Geometry check sheet. Reference: the model listing, model coordinates, mm. Face numbers are marked on the shaded views. A direction names the side the tool comes from. Give positions to 0.01 mm unless a question says otherwise; leave off trailing zeros. Loops run counter-clockwise (first coordinate to the right, second up) from the corner with the lowest first, then second, coordinate; pieces in that order, holes last. Notation, with made-up numbers: (-13, -6) -> (33, -6) arc R9 ccw to (33, 4) -> close; hole circle Ø5 at (75, 16.25). An arc over 180 degrees is marked (long way). Answer as a JSON object with one key per item and string values.
from build123d import *

# Parameters (mm, degrees)
SKETCH1_W           = 10
SKETCH1_H           = 10
BOSS_EXTRUDE1_DEPTH = 5
CUT_EXTRUDE1_START  = 1.25
CUT_EXTRUDE1_DEPTH  = 2.5
SKETCH2_R           = 1.6
CUT_EXTRUDE2_DEPTH  = 6


with BuildPart() as part:
    # Sketch1 → Boss-Extrude1 (new body)
    with BuildSketch(Plane.XY):
        Rectangle(SKETCH1_W, SKETCH1_H)
        Polygon((2.975, 1.717617051), (0, 3.435234102), (-2.975, 1.717617051), (-2.975, -1.717617051), (0, -3.435234102), (2.975, -1.717617051), align=None, mode=Mode.SUBTRACT)
        Polygon((2.975, -1.717617051), (2.975, 1.717617051), (0, 3.435234102), (-2.975, 1.717617051), (-2.975, -1.717617051), (0, -3.435234102), align=None)
    extrude(amount=BOSS_EXTRUDE1_DEPTH)

    # Sketch1_3 → Cut-Extrude1 (cut)
    with BuildSketch(Plane.XY.offset(CUT_EXTRUDE1_START)):
        Polygon((2.975, -1.717617051), (2.975, 1.717617051), (0, 3.435234102), (-2.975, 1.717617051), (-2.975, -1.717617051), (0, -3.435234102), align=None)
    extrude(amount=CUT_EXTRUDE1_DEPTH, mode=Mode.SUBTRACT)

    # Sketch2 → Cut-Extrude2 (cut, through all)
    with BuildSketch(Plane.XY.offset(5)):
        Circle(SKETCH2_R)
    extrude(amount=-CUT_EXTRUDE2_DEPTH, mode=Mode.SUBTRACT)


solid = part.part
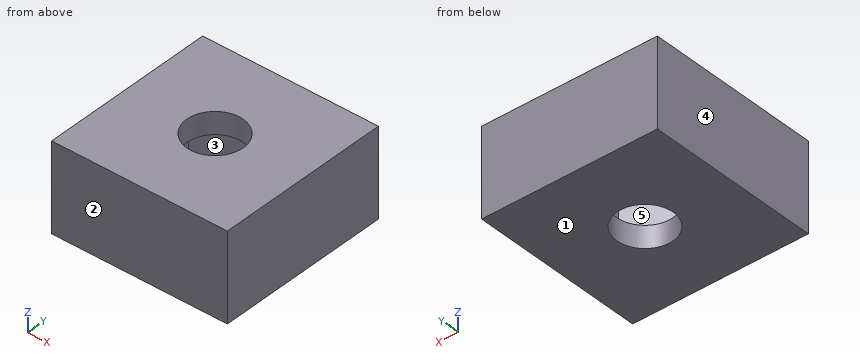
1) Draft check along Y on the marked faces 1, 2 and 3. Enter one of: pulls with the +Y half, pulls with the -Y half, needs draft (parallel to the pull), parting line crosses it, or undercut.
Geometry check:
{"face 1": "needs draft", "face 2": "pulls with the -Y half", "face 3": "undercut"}
2) Section check C-C on x = 0.75. Record the cut outline in (y, z), plus the area to 3 significant figures.
Geometry check:
{"outline": "(-5, 0) -> (-1.41, 0) -> (-1.41, 1.25) -> (-3, 1.25) -> (-3, 3.75) -> (-1.41, 3.75) -> (-1.41, 5) -> (-5, 5) -> close; (1.41, 0) -> (5, 0) -> (5, 5) -> (1.41, 5) -> (1.41, 3.75) -> (3, 3.75) -> (3, 1.25) -> (1.41, 1.25) -> close", "area": "27.9 mm2"}
3) Section check B-B on y = 0.25. Record the cut outline in (x, z) (3 decimals), plus the area to 3 significant figures.
Geometry check:
{"outline": "(-5, 0) -> (-1.58, 0) -> (-1.58, 1.25) -> (-2.975, 1.25) -> (-2.975, 3.75) -> (-1.58, 3.75) -> (-1.58, 5) -> (-5, 5) -> close; (1.58, 0) -> (5, 0) -> (5, 5) -> (1.58, 5) -> (1.58, 3.75) -> (2.975, 3.75) -> (2.975, 1.25) -> (1.58, 1.25) -> close", "area": "27.2 mm2"}
4) Material ranges on line 1 along X through (y, z) = (0, 2.25) (3 decimals); line 2 along Z through (x, y) = (0.5, -2.5); line 3 along Y through (x, z) = (0, 4.6), recorded low to high. Write a range as from..to.
Geometry check:
{"line 1": "x = -5..-2.975, 2.975..5", "line 2": "z = 0..1.25, 3.75..5", "line 3": "y = -5..-1.6, 1.6..5"}
5) Section check A-A on z = 3. Record the cut outline in (x, y) (3 decimals).
Geometry check:
{"outline": "(-5, -5) -> (5, -5) -> (5, 5) -> (-5, 5) -> close; hole (-2.975, -1.718) -> (0, -3.435) -> (2.975, -1.718) -> (2.975, 1.718) -> (0, 3.435) -> (-2.975, 1.718) -> close"}
6) Tool access check on the marked faces 4 and 5. Record the directions out of +Z, -Z, +X, -X, +Y, -Y that give a thin tool (end or side, any length) a straight path to the whole face; none if there is none.
Geometry check:
{"face 4": "+Z, -Z, -X, +Y, -Y", "face 5": "none"}
7) Section check D-D on y = -2.5. Record the cut outline in (x, z).
Geometry check:
{"outline": "(-5, 0) -> (5, 0) -> (5, 5) -> (-5, 5) -> close; hole (-1.62, 1.25) -> (1.62, 1.25) -> (1.62, 3.75) -> (-1.62, 3.75) -> close"}
